Work out the finished part from the listing and answer in its coordinate system (mm). Face numbers are marked on the shaded views. A direction names the side the tool comes from. Give positions to 0.01 mm unless a question says otherwise; leave off trailing zeros. Order: outer loops, then holes, each group sorted by start corner. A loop starts at its lowest first (then second) coordinate and runs counter-clockwise, first axis right, second up. Notation, with made-up numbers: M -2.75,41 L 41.25,41 A7 ccw 41.25,51 Z; hole C -38,-6 d1. An arc over 180 degrees is marked long. One line per item, written item: value.
from build123d import *

# Parameters (mm, degrees)
SKETCH1_W           = 8
SKETCH1_H           = 8
BOSS_EXTRUDE1_DEPTH = 2
FILLET2_R           = 0.5


with BuildPart() as part:
    # Sketch1 → Boss-Extrude1 (new body)
    with BuildSketch(Plane(origin=(0, 0, 0), x_dir=(1, 0, 0), z_dir=(0, 1, 0))):
        Rectangle(SKETCH1_W, SKETCH1_H)
        with BuildLine():
            ThreePointArc((-5, 0), (-5.034074174, 0.258819045), (-5.133974596, 0.5))
            Line((-5.133974596, 0.5), (-6, 0.5))
            Line((-6, 0.5), (-6, -0.5))
            Line((-6, -0.5), (-5.133974596, -0.5))
            ThreePointArc((-5.133974596, -0.5), (-5.034074174, -0.258819045), (-5, 0))
        make_face()
        with BuildLine():
            Line((-6, 0.5), (-5.133974596, 0.5))
            ThreePointArc((-5.133974596, 0.5), (-7, 0), (-5.133974596, -0.5))
            Line((-5.133974596, -0.5), (-6, -0.5))
            Line((-6, -0.5), (-6, 0.5))
        make_face()
        with BuildLine():
            Line((-4, -0.5), (-4, 0.5))
            Line((-4, 0.5), (-5.133974596, 0.5))
            ThreePointArc((-5.133974596, 0.5), (-5.034074174, 0.258819045), (-5, 0))
            ThreePointArc((-5, 0), (-5.034074174, -0.258819045), (-5.133974596, -0.5))
            Line((-5.133974596, -0.5), (-4, -0.5))
        make_face()
        with BuildLine():
            Line((0, 5), (0, 4))
            Line((0, 4), (0.5, 4))
            Line((0.5, 4), (0.5, 5.133974596))
            ThreePointArc((0.5, 5.133974596), (0.258819045, 5.034074174), (0, 5))
        make_face()
        with BuildLine():
            Line((-0.5, 5.133974596), (-0.5, 4))
            Line((-0.5, 4), (0, 4))
            Line((0, 4), (0, 5))
            ThreePointArc((0, 5), (-0.258819045, 5.034074174), (-0.5, 5.133974596))
        make_face()
        with BuildLine():
            Line((-0.5, 6), (-0.5, 5.133974596))
            ThreePointArc((-0.5, 5.133974596), (-0.258819045, 5.034074174), (0, 5))
            Line((0, 5), (0, 6))
            Line((0, 6), (-0.5, 6))
        make_face()
        with BuildLine():
            Line((0, 6), (0, 5))
            ThreePointArc((0, 5), (0.258819045, 5.034074174), (0.5, 5.133974596))
            Line((0.5, 5.133974596), (0.5, 6))
            Line((0.5, 6), (0, 6))
        make_face()
        with BuildLine():
            ThreePointArc((1, 6), (-0.5, 6.866025404), (-0.5, 5.133974596))
            Line((-0.5, 5.133974596), (-0.5, 6))
            Line((-0.5, 6), (0, 6))
            Line((0, 6), (0.5, 6))
            Line((0.5, 6), (0.5, 5.133974596))
            ThreePointArc((0.5, 5.133974596), (0.866025404, 5.5), (1, 6))
        make_face()
        with BuildLine():
            ThreePointArc((7, 0), (6.258819045, 0.965925826), (5.133974596, 0.5))
            Line((5.133974596, 0.5), (6, 0.5))
            Line((6, 0.5), (6, -0.5))
            Line((6, -0.5), (5.133974596, -0.5))
            ThreePointArc((5.133974596, -0.5), (6.258819045, -0.965925826), (7, 0))
        make_face()
        with BuildLine():
            Line((6, 0.5), (5.133974596, 0.5))
            ThreePointArc((5.133974596, 0.5), (5, 0), (5.133974596, -0.5))
            Line((5.133974596, -0.5), (6, -0.5))
            Line((6, -0.5), (6, 0.5))
        make_face()
        with BuildLine():
            ThreePointArc((0.5, -5.133974596), (0, -5), (-0.5, -5.133974596))
            Line((-0.5, -5.133974596), (-0.5, -6))
            Line((-0.5, -6), (0.5, -6))
            Line((0.5, -6), (0.5, -5.133974596))
        make_face()
        with BuildLine():
            Line((-0.5, -6), (-0.5, -5.133974596))
            ThreePointArc((-0.5, -5.133974596), (-0.5, -6.866025404), (1, -6))
            ThreePointArc((1, -6), (0.866025404, -5.5), (0.5, -5.133974596))
            Line((0.5, -5.133974596), (0.5, -6))
            Line((0.5, -6), (-0.5, -6))
        make_face()
        with BuildLine():
            Line((0.5, -4), (-0.5, -4))
            Line((-0.5, -4), (-0.5, -5.133974596))
            ThreePointArc((-0.5, -5.133974596), (0, -5), (0.5, -5.133974596))
            Line((0.5, -5.133974596), (0.5, -4))
        make_face()
        with BuildLine():
            Line((5.133974596, 0.5), (4, 0.5))
            Line((4, 0.5), (4, -0.5))
            Line((4, -0.5), (5.133974596, -0.5))
            ThreePointArc((5.133974596, -0.5), (5, 0), (5.133974596, 0.5))
        make_face()
    extrude(amount=BOSS_EXTRUDE1_DEPTH)

    # Fillet2
    fillet2_edges = [part.edges().sort_by_distance(p)[0] for p in [
        (0.5, 1, -4),
        (4, 1, -0.5),
        (5.133974596, 1, -0.5),
        (5.133974596, 1, 0.5),
        (4, 1, 0.5),
        (0.5, 1, 4),
        (0.5, 1, 5.133974596),
        (-0.5, 1, 5.133974596),
        (-0.5, 1, 4),
        (-4, 1, 0.5),
        (-5.133974596, 1, 0.5),
        (-5.133974596, 1, -0.5),
        (-4, 1, -0.5),
        (-0.5, 1, -4),
        (-0.5, 1, -5.133974596),
        (0.5, 1, -5.133974596),
    ]]
    fillet(fillet2_edges, radius=FILLET2_R)


solid = part.part
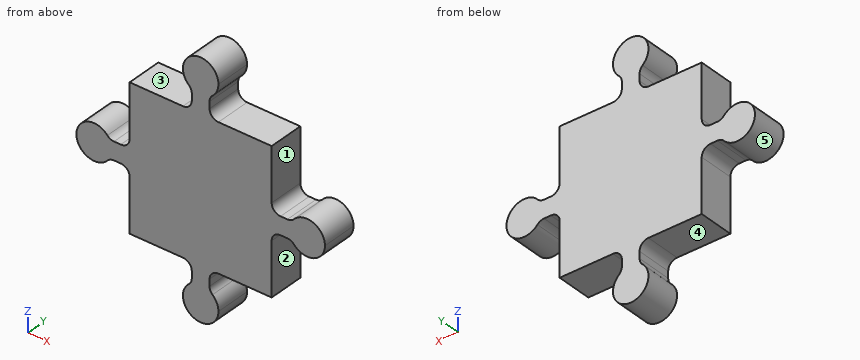
(1) Find the intervals of material crossed by probe 1 along Z at (x, y) = (-0.75, 1.5); probe 2 along Z at (x, y) = (-1.25, 1.55), in increasing order. Write a range as from..to.
Findings:
probe 1: z = -6.66..-5.34, -4.07..4.07, 5.34..6.66
probe 2: z = -4..4
(2) Section A-A, the plane x = 3.75 is taken. Give the vertices of the cut face in (y, z), then the cut area to 3 significant figures.
Findings:
outline: M 0,-4 L 2,-4 L 2,4 L 0,4 Z
area: 16.0 mm^2
(3) Which of the six approach directions +Z, -Z, +X, -X, +Y, -Y give full straight-line access (tool end or side, diameter ignored) to the marked faces 1, 2, 3, 4 and 5?
Findings:
face 1: +Z, +X, +Y, -Y
face 2: -Z, +X, +Y, -Y
face 3: +Z, -X, +Y, -Y
face 4: -Z, -X, +Y, -Y
face 5: +Y, -Y
(4) Given P1, Ø4, axis at x = 5, z = -4.5, coming from the +Y side; P2, Ø0.6, axis at y = 1.5, z = 2, coming from the +X side; P3, Ø1, axis at x = -2.5, y = 1, coming from the +Z side; P4, Ø0.6, axis at x = -3, y = 1, coming from the -Z side, each flat-ended and moving along its own axis, determine where each tip first touches the part or whether it passes through.
Findings:
P1: stops at y = 2
P2: stops at x = 4
P3: stops at z = 4
P4: stops at z = -4
